The model under review builds one solid part; all positions refer to its coordinate system, in mm. A direction names the side the tool comes from. Coordinates: 2 decimals unless noted, no trailing zeros. Order: outer loops, then holes, each group sorted by start corner. A loop starts at its lowest first (then second) coordinate and runs counter-clockwise, first axis right, second up. Notation, with made-up numbers: M 0.5,39 L 22.5,39 A30 ccw 22.5,64 Z; hole C 78,-30 d3. An arc over 180 degrees is marked long. Answer as CSV lines item,"result". Start each with the question number.
Q1. Wall thickness on L1, parallel to Y at x = 0, z = -31 (3 decimals); L2, parallel to Y at x = 6, z = -5.5; L3, parallel to Y at x = 0, z = -9.5 (1 decimal): over which ranges is each line inside the solid? List them lowest first. Write a range as [from, to].
Q2. Consider section B-B on z = 21. Write out the cut boundary in (x, y).
Q3. Consider section C-C on z = 7. Write out the cut boundary in (x, y) (1 decimal), and give its area (3 significant figures).
Q4. Consider section A-A on z = -22. State how many separate pieces and enclosed holes the cut face has, and give its area (3 significant figures).
Q5. Machinability: for faces 1 (the face through (-0.9, 16.2, 24)), 2 (the face through (-0.1, -16.2, 22)), 3 (the face through (-11, 11, 23)), which of the approach directions +Z, -Z, +X, -X, +Y, -Y give a long, thin tool a straight path to every point of the face, cutting with its end or side? Answer none if there is none.
Q6. For P1, Ø1.6, axis at y = -12, z = 23, coming from the +X side; P2, Ø10, axis at x = 0, y = 0, coming from the +Z side; P3, Ø4, axis at x = 3, y = 11, coming from the +Z side; P4, Ø4, axis at y = 13.5, z = -16, coming from the -X side, all flat-tipped, find the tip position at first contact; note any pin that passes through.
Q7. The part is to be moulded in two halves that separate along Z. For faces 4 (the face through (-1.172, 8.923, -11.745)), 5 (the face through (-8.5, 12, 23)), 6 (the face through (-6, 13, 26)), say which applies: +Z half, -Z half, draft (parallel to the pull), parting line (faces both ways), or undercut.
from build123d import *

# Parameters (mm, degrees)
SKETCH1_R                = 15.5
BOSS_EXTRUDE5_DEPTH      = 26
SKETCH3_R                = 5.625
CUT_EXTRUDE2_DEPTH       = 35.007352146
CUT_EXTRUDE3_DEPTH       = 28
CUT_EXTRUDE3_DEPTH_BACK  = 20
SKETCH4_R                = 11.1125
CUT_EXTRUDE6_START       = 6
SKETCH7_R                = 11
SKETCH7_R_2              = 9
CUT_EXTRUDE6_DEPTH       = 2
BOSS_EXTRUDE8_DEPTH      = 6
BOSS_EXTRUDE8_DEPTH_BACK = 2
BOSS_EXTRUDE8_START      = 20
SKETCH12_R               = 17
CUT_EXTRUDE10_START      = 18
SKETCH13_R               = 11
CUT_EXTRUDE10_DEPTH      = 18.411862419
FILLET2_R                = 2
CUT_EXTRUDE11_START      = 26
SKETCH14_R               = 14
CUT_EXTRUDE11_DEPTH      = 6
SKETCH15_R               = 0.5
CUT_EXTRUDE14_DEPTH      = 36.411862419
SKETCH18_W               = 2.5
SKETCH18_H               = 2
CUT_EXTRUDE15_DEPTH      = 20
CUT_EXTRUDE16_DEPTH      = 2
BOSS_EXTRUDE9_START      = 33
SKETCH26_R               = 15.5
SKETCH26_R_2             = 5.625
SKETCH26_R_3             = 0.5
BOSS_EXTRUDE9_DEPTH      = 33
SKETCH27_R               = 11.1125
CUT_EXTRUDE17_DEPTH      = 33
BOSS_EXTRUDE10_START     = -35
SKETCH24_R               = 9
SKETCH24_R_2             = 5.625
BOSS_EXTRUDE10_DEPTH     = 35


with BuildPart() as part:
    # Sketch1 → Boss-Extrude5 (new body)
    with BuildSketch(Plane.XY):
        Circle(SKETCH1_R)
    extrude(amount=BOSS_EXTRUDE5_DEPTH)

    # Sketch3 → Cut-Extrude2 (cut, through all)
    with BuildSketch(Plane.XY.offset(26)):
        Circle(SKETCH3_R)
    extrude(amount=-CUT_EXTRUDE2_DEPTH, mode=Mode.SUBTRACT)

    # Sketch4 → Cut-Extrude3 (cut, two sides: drawn at the far end of the back side and taken through both)
    with BuildSketch(Plane.XY.offset(26).offset(-CUT_EXTRUDE3_DEPTH_BACK)):
        Circle(SKETCH4_R)
    extrude(amount=CUT_EXTRUDE3_DEPTH + CUT_EXTRUDE3_DEPTH_BACK, mode=Mode.SUBTRACT)

    # Sketch7 → Cut-Extrude6 (cut)
    with BuildSketch(Plane.XY.offset(CUT_EXTRUDE6_START)):
        Circle(SKETCH7_R)
        Circle(SKETCH7_R_2, mode=Mode.SUBTRACT)
    extrude(amount=-CUT_EXTRUDE6_DEPTH, mode=Mode.SUBTRACT)

    # Sketch12 → Boss-Extrude8 (add, two sides: drawn at the far end of the back side and taken through both)
    with BuildSketch(Plane.XY.offset(BOSS_EXTRUDE8_START - BOSS_EXTRUDE8_DEPTH_BACK)):
        Circle(SKETCH12_R)
    extrude(amount=BOSS_EXTRUDE8_DEPTH + BOSS_EXTRUDE8_DEPTH_BACK)

    # Sketch13 → Cut-Extrude10 (cut, through all)
    with BuildSketch(Plane.XY.offset(CUT_EXTRUDE10_START)):
        Circle(SKETCH13_R)
    extrude(amount=CUT_EXTRUDE10_DEPTH, mode=Mode.SUBTRACT)

    # Fillet2
    # the kernel refuses this fillet: 2 mm, written as the material it adds along each edge
    with BuildSketch(Plane(origin=(0, 0, 18), x_dir=(1, 0, 0), z_dir=(0, 1, 0))) as fillet2_piece_1:
        with BuildLine():
            CenterArc((17.5, 1.936491673), FILLET2_R, 180, 75.522487814)
            Line((17, 0), (16.99, -0.038729833))
            ThreePointArc((16.99, -0.038729833), (16.25, -0.04), (15.5, -0.04))
            Line((15.5, -0.04), (15.46, 0))
            Line((15.46, 0), (15.46, 1.936491673))
            Line((15.46, 1.936491673), (15.5, 1.936491673))
        make_face()
    revolve(axis=Axis((0, 0, 18), (0, 0, -1)))

    # Sketch14 → Cut-Extrude11 (cut)
    with BuildSketch(Plane.XY.offset(CUT_EXTRUDE11_START)):
        Circle(SKETCH14_R)
    extrude(amount=-CUT_EXTRUDE11_DEPTH, mode=Mode.SUBTRACT)

    # Sketch15 → Cut-Extrude14 (cut, through all)
    with BuildSketch(Plane.XY):
        with Locations((0, 10)):
            Circle(SKETCH15_R)
        with Locations((0, -10)):
            Circle(SKETCH15_R)
        with Locations((10, 0)):
            Circle(SKETCH15_R)
        with Locations((-10, 0)):
            Circle(SKETCH15_R)
    extrude(amount=CUT_EXTRUDE14_DEPTH, mode=Mode.SUBTRACT)

    # Sketch18 → Cut-Extrude15 (cut, symmetric)
    with BuildSketch(Plane(origin=(0, 0, 0), x_dir=(1, 0, 0), z_dir=(0, 1, 0))):
        with Locations((-9.75, -23)):
            Rectangle(SKETCH18_W, SKETCH18_H)
        with Locations((9.75, -23)):
            Rectangle(SKETCH18_W, SKETCH18_H)
    extrude(amount=CUT_EXTRUDE15_DEPTH, both=True, mode=Mode.SUBTRACT)

    # Sketch23 → Cut-Extrude16 (cut)
    with BuildSketch(Plane(origin=(0, 0, 24), x_dir=(-1, 0, 0), z_dir=(0, 0, -1))):
        with BuildLine():
            Line((9.719197711, 13.947659153), (9.147480199, 13.127208615))
            ThreePointArc((9.147480199, 13.127208615), (0, 16), (-9.147480199, 13.127208615))
            Line((-9.147480199, 13.127208615), (-9.719197711, 13.947659153))
            ThreePointArc((-9.719197711, 13.947659153), (0, 17), (9.719197711, 13.947659153))
        make_face()
        with BuildLine():
            Line((-9.147480199, -13.127208615), (-9.719197711, -13.947659153))
            ThreePointArc((-9.719197711, -13.947659153), (0, -17), (9.719197711, -13.947659153))
            Line((9.719197711, -13.947659153), (9.147480199, -13.127208615))
            ThreePointArc((9.147480199, -13.127208615), (0, -16), (-9.147480199, -13.127208615))
        make_face()
    extrude(amount=CUT_EXTRUDE16_DEPTH, mode=Mode.SUBTRACT)

    # Sketch26 → Boss-Extrude9 (add)
    with BuildSketch(Plane(origin=(0, 0, 0), x_dir=(-1, 0, 0), z_dir=(0, 0, -1)).offset(BOSS_EXTRUDE9_START)):
        Circle(SKETCH26_R)
        with Locations(Location((0, 0, 0), (0, 0, 180))):
            Circle(SKETCH26_R_2, mode=Mode.SUBTRACT)
        with Locations((-10, 0)):
            Circle(SKETCH26_R_3, mode=Mode.SUBTRACT)
        with Locations((0, 10)):
            Circle(SKETCH26_R_3, mode=Mode.SUBTRACT)
        with Locations((10, 0)):
            Circle(SKETCH26_R_3, mode=Mode.SUBTRACT)
        with Locations((0, -10)):
            Circle(SKETCH26_R_3, mode=Mode.SUBTRACT)
    extrude(amount=-BOSS_EXTRUDE9_DEPTH)

    # Sketch27 → Cut-Extrude17 (cut, symmetric)
    with BuildSketch(Plane.XY.offset(4)):
        Circle(SKETCH27_R)
    extrude(amount=CUT_EXTRUDE17_DEPTH, both=True, mode=Mode.SUBTRACT)

    # Sketch24 → Boss-Extrude10 (add)
    with BuildSketch(Plane.XY.offset(6).offset(BOSS_EXTRUDE10_START)):
        Circle(SKETCH24_R)
        Circle(SKETCH24_R_2, mode=Mode.SUBTRACT)
    extrude(amount=BOSS_EXTRUDE10_DEPTH)


solid = part.part
Evaluation:
1,L1,"y = [-15.5, -10.5], [-9.5, -5.625], [5.625, 9.5], [10.5, 15.5]"
1,L2,"y = [-14.29, -9.35], [-6.71, 6.71], [9.35, 14.29]"
1,L3,"y = [-15.5, -11.1], [-9, -5.6], [5.6, 9], [11.1, 15.5]"
2,outline,"C 0,0 d34; hole C 0,0 d28"
3,outline,"C 0,0 d31; hole C 0,0 d22.2"
3,area,"367 mm²"
4,separate pieces,"2"
4,enclosed holes,"2"
4,area,"522 mm²"
5,face 1,"+Y"
5,face 2,"-Y"
5,face 3,"+Y, -Y"
6,P1,"stops at x = 12.79"
6,P2,"passes through"
6,P3,"stops at z = 20"
6,P4,"stops at x = -10.39"
7,face 4,"draft"
7,face 5,"undercut"
7,face 6,"+Z half"
